Autodesk Fusion 360 part; units mm, degrees
sketch "草图1" plane through (0, 0, 13.3714) normal (0, 0, 1) x (-1, 0, 0)
  line L0 (10.9987, -232.8503) -> (25.9987, -232.8503)
  line L1 (25.9987, -232.8503) -> (25.9987, -126.3503)
  line L2 (25.9987, -126.3503) -> (-124.0013, -126.3503)
  line L3 (-124.0013, -126.3503) -> (-124.0013, -232.8503)
  line L4 (-124.0013, -232.8503) -> (-109.0013, -232.8503)
  line L5 (-109.0013, -232.8503) -> (-109.0013, -225.3503)
  line L6 (-109.0013, -225.3503) -> (-103.0013, -225.3503)
  line L7 (-103.0013, -225.3503) -> (-103.0013, -232.8503)
  line L8 (-103.0013, -232.8503) -> (-52.0013, -232.8503)
  line L9 (-52.0013, -232.8503) -> (-52.0013, -225.3503)
  line L10 (-52.0013, -225.3503) -> (-46.0013, -225.3503)
  line L11 (-46.0013, -225.3503) -> (-46.0013, -232.8503)
  line L12 (-46.0013, -232.8503) -> (4.9987, -232.8503)
  line L13 (4.9987, -232.8503) -> (4.9987, -225.3503)
  line L14 (4.9987, -225.3503) -> (10.9987, -225.3503)
  line L15 (10.9987, -225.3503) -> (10.9987, -232.8503)
  line L16 (-114.0013, -225.3503) -> (-127.4522, -225.3503)
  line L17 (-127.4522, -225.3503) -> (-127.4522, -236.557)
  line L18 (-127.4522, -236.557) -> (-114.0013, -236.557)
  line L19 (-114.0013, -236.557) -> (-114.0013, -225.3503)
  line L20 (-98.0013, -225.3503) -> (-57.0013, -225.3503)
  line L21 (-57.0013, -225.3503) -> (-57.0013, -239)
  line L22 (-57.0013, -239) -> (-98.0013, -239)
  line L23 (-98.0013, -239) -> (-98.0013, -225.3503)
  line L24 (-41.0013, -225.3503) -> (-0.0013, -225.3503)
  line L25 (-0.0013, -225.3503) -> (-0.0013, -240)
  line L26 (-0.0013, -240) -> (-41.0013, -240)
  line L27 (-41.0013, -240) -> (-41.0013, -225.3503)
  line L28 (15.9987, -225.3503) -> (29.1278, -225.3503)
  line L29 (29.1278, -225.3503) -> (29.1278, -239)
  line L30 (29.1278, -239) -> (15.9987, -239)
  line L31 (15.9987, -239) -> (15.9987, -225.3503)
  dimension "d1" = 5
  dimension "d2" = 5
  dimension "d3" = 5
  dimension "d4" = 5
  dimension "d5" = 5
  dimension "d6" = 5
sketch "草图2" plane through (150, 0, 0) normal (1, 0, 0) x (0, 1, 0)
  line L0 (0, 100) -> (109, 100)
  line L1 (109, 100) -> (109, 106)
  line L2 (109, 106) -> (0, 106)
  line L3 (0, 106) -> (0, 100)
  circle A0 centre (106, 103) radius 2
  dimension "d7" = 4
  dimension "d8" = 3
  dimension "d9" = 3
sketch "草图3" plane through (0, 0, 100) normal (0, 0, 1) x (-1, 0, 0)
  line L0 (-3, -29) -> (0, -29)
  line L1 (0, -29) -> (0, 0)
  line L2 (0, 0) -> (-63, 0)
  line L3 (-63, 0) -> (-63, -3)
  line L4 (-63, -3) -> (-3, -3)
  line L5 (-3, -3) -> (-3, -29)
  line L6 (0, -109) -> (-150, -109)
  line L7 (-150, -109) -> (-150, 0)
  line L8 (-150, 0) -> (0, 0)
  line L9 (0, 0) -> (0, -109)
  dimension "d10" = 150
  dimension "d11" = 109
sketch "草图4" plane through (0, 0, 106) normal (0, 0, 1) x (-1, 0, 0)
  line L0 (0, 0) -> (-150, 0)
  line L1 (-150, 0) -> (-150, -109)
  line L2 (-150, -109) -> (0, -109)
  line L3 (0, -109) -> (0, 0)
  line L4 (-135, -99) -> (-129, -99)
  line L5 (-129, -99) -> (-129, -109)
  line L6 (-129, -109) -> (-135, -109)
  line L7 (-135, -109) -> (-135, -99)
  line L8 (-78, -99) -> (-72, -99)
  line L9 (-72, -99) -> (-72, -109)
  line L10 (-72, -109) -> (-78, -109)
  line L11 (-78, -109) -> (-78, -99)
  line L12 (-21, -99) -> (-15, -99)
  line L13 (-15, -99) -> (-15, -109)
  line L14 (-15, -109) -> (-21, -109)
  line L15 (-21, -109) -> (-21, -99)
  dimension "d12" = 6
  dimension "d13" = 10
  dimension "d14" = 15
  dimension "d15" = 6
  dimension "d16" = 10
  dimension "d17" = 6
  dimension "d18" = 10
  dimension "d19" = 72
  dimension "d20" = 15
extrude "拉伸1" add sketch "草图3" along normal blind 6
extrude "拉伸2" cut sketch "草图4" against normal blind 10 contours L2 L12 L13 L14 L15 | L2 L4 L5 L6 L7 | L2 L8 L9 L10 L11
extrude "拉伸3" cut sketch "草图2" against normal blind 170 contours A0
fillet "圆角1" radius 2.5 4 edges at (142.5, 109, 106) (103.5, 109, 106) (46.5, 109, 106) (7.5, 109, 106)
extrude "拉伸4" cut sketch "草图1" against normal blind 25 contours L0 L1 L28 L31 | L0 L1 L28 L29 L30 L31 | L12 L25 L26 L27 | L12 L24 L25 L27 | L3 L4 L16 L19 | L3 L4 L16 L17 L18 L19 | L8 L21 L22 L23 | L8 L20 L21 L23
Geometry: final body of the model. Coordinates: model frame, mm. A direction names the side the tool comes from. Give positions to 0.01 mm unless a question says otherwise; leave off trailing zeros. Write each loop counter-clockwise with the first axis right and the second up, starting at its lowest first coordinate (ties: lowest second). Pieces come first, ordered by that corner, then holes. Notation, with made-up numbers: (57.25, 37.5) - (83.25, 37.5) arc R9 ccw to (83.25, 53.5) - close; hole circle Ø11 at (54.5, 43). An arc over 180 degrees is marked (long way). Return JSON: item names as keys, results as strings. Group by question number.
1) Section A-A on x = 48.5. Return the cut outline in (y, z).
2) Mould query, pull axis Z, two halves, no side actions, for faces 1 (the cylindrical face through (47, 106, 105)), 2 (the flat face through (135, 103, 103)), 3 (the flat face through (76, 54, 100)). Classes: released by +Z, released by -Z, zero draft, split by the parting line, or undercut.
3) Set-up query: faces 4 (the cylindrical face through (8, 106, 105)), 5 (the flat face through (78, 103, 103)). Return all of +Z, -Z, +X, -X, +Y, -Y with unobstructed straight access to the full face (end or side cutting, diameter ignored); none if empty.
4) Line query: line 1 (Z direction, x = 111.5, y = 106); line 2 (Y direction, x = 68.5, z = 103.55); line 3 (Y direction, x = 70, z = 101.3). Output: solid intervals per line, ascending.
5) Section B-B on x = 18.5. Return the cut outline in (y, z).
6) First-contact query: P1, Ø3, axis at x = 129, z = 103.5, coming from the -Y side; P2, Ø1.8, axis at x = 74.5, z = 104, coming from the +Y side. Flat tips, straight axial feed; report the tip coordinate or a pass-through.
Filled in:
{
 "1": {"outline": "(0, 100) - (109, 100) - (109, 103.5) arc R2.5 ccw to (106.5, 106) - (0, 106) - close; hole circle Ø4 at (106, 103)"},
 "2": {"face 1": "undercut", "face 2": "zero draft", "face 3": "released by -Z"},
 "3": {"face 4": "+X, -X", "face 5": "+Z, -Z, +Y"},
 "4": {"line 1": "z = 100 to 101, 105 to 106", "line 2": "y = 0 to 104.08, 107.92 to 109", "line 3": "y = 0 to 104.95, 107.05 to 109"},
 "5": {"outline": "(0, 100) - (99, 100) - (99, 106) - (0, 106) - close"},
 "6": {"P1": "stops at y = 0", "P2": "stops at y = 99"}
}
